from build123d import *

# Parameters (mm, degrees)
AUFSATZ_LINEAR_AUSTRAGEN1_DEPTH = 30
F_3_0_3_DURCHMESSER_BOHRUNG1_D  = 3
SCHNITT_LINEAR_AUSTRAGEN1_DEPTH = 4


with BuildPart() as part:
    # Skizze1 → Aufsatz-Linear austragen1 (new body)
    with BuildSketch(Plane.XY):
        with BuildLine():
            Line((-63.596153483, 25.865230167), (-58.344999569, 25.865230167))
            ThreePointArc((-58.344999569, 25.865230167), (-48.596153483, 34.665230167), (-38.847307398, 25.865230167))
            Line((-38.847307398, 25.865230167), (-34.847307398, 25.865230167))
            Line((-34.847307398, 25.865230167), (-34.176711032, 25.865230167))
            Line((-34.176711032, 25.865230167), (-33.778455993, 25.865230167))
            Line((-33.778455993, 25.865230167), (-33.778455993, 37.365230166))
            Line((-33.778455993, 37.365230166), (-34.847307398, 37.365230166))
            Line((-34.847307398, 37.365230166), (-48.596153483, 37.365230166))
            Line((-48.596153483, 37.365230166), (-63.596153483, 37.365230166))
            Line((-63.596153483, 37.365230166), (-63.596153483, 25.865230167))
        make_face()
    extrude(amount=-AUFSATZ_LINEAR_AUSTRAGEN1_DEPTH)

    # Ø3.0 (3) Durchmesser Bohrung1 (through all)
    with Locations(Plane(origin=(0, 37.365230166, 0), x_dir=(1, 0, 0), z_dir=(0, 1, 0))):
        with Locations((-36.847307398, 5), (-60.344999569, 5), (-60.344999569, 25), (-36.847307398, 25)):
            Hole(F_3_0_3_DURCHMESSER_BOHRUNG1_D / 2)

    # Skizze4 → Schnitt-Linear austragen1 (cut)
    with BuildSketch(Plane(origin=(0, 37.365230166, 0), x_dir=(1, 0, 0), z_dir=(0, 1, 0))):
        Polygon((-39.747307398, 26.674315781), (-39.747307398, 23.325684219), (-36.847307398, 21.651368439), (-33.947307398, 23.325684219), (-33.947307398, 26.674315781), (-36.847307398, 28.348631561), align=None)
        Polygon((-60.344999569, 28.348631561), (-63.244999569, 26.674315781), (-63.244999569, 23.325684219), (-60.344999569, 21.651368439), (-57.444999569, 23.325684219), (-57.444999569, 26.674315781), align=None)
        Polygon((-63.244999569, 6.674315781), (-63.244999569, 3.325684219), (-60.344999569, 1.651368439), (-57.444999569, 3.325684219), (-57.444999569, 6.674315781), (-60.344999569, 8.348631561), align=None)
        Polygon((-36.847307398, 8.348631561), (-39.747307398, 6.674315781), (-39.747307398, 3.325684219), (-36.847307398, 1.651368439), (-33.947307398, 3.325684219), (-33.947307398, 6.674315781), align=None)
    extrude(amount=-SCHNITT_LINEAR_AUSTRAGEN1_DEPTH, mode=Mode.SUBTRACT)


solid = part.part
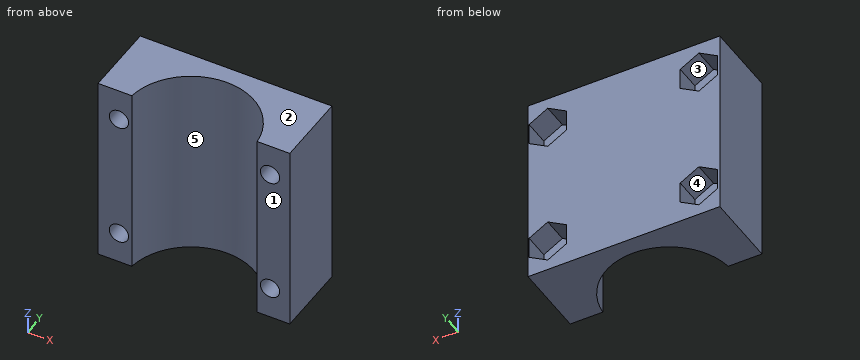
For this review, take the finished solid that the model builds, in its own axes (mm). Face numbers are marked on the shaded views. A direction names the side the tool comes from. Give positions to 0.01 mm unless a question says otherwise; leave off trailing zeros. Loops run counter-clockwise (first coordinate to the right, second up) from the corner with the lowest first, then second, coordinate; pieces in that order, holes last.
Item 1: Take a section at D-D, the plane x = -39.25. State the section outline as (y, z) points.
Item 2: Draft analysis for pull direction Z (two halves, no side actions). For the marked faces 1, 2 and 3, state which applies: +Z half, -Z half, draft (parallel to the pull), parting line (faces both ways), or undercut.
Item 3: Tool access review of the marked faces 4 and 5: name each direction out of +Z, -Z, +X, -X, +Y, -Y from which nothing blocks a thin tool from reaching the whole face with its end or side.
Item 4: For line 1 along Z through (x, y) = (-37, 27.25); line 2 along X through (y, z) = (30.25, -25) (3 decimals); line 3 along X through (y, z) = (32, -26), list the stretches that pass through material, from the lowest coordinate up.
Item 5: Insertion check: pin 1 (3 mm diameter, centred on x = -60.5, z = -24, fed in from +Y). The pin has a flat end and moves straight along its axis. Give the tip position at first contact, or say it passes through.
Item 6: Take a section at C-C, the plane z = -12. State the section outline as (x, y) points (3 decimals), and give its area (3 significant figures).
Item 7: Take a section at A-A, the plane z = -25. State the section outline as (x, y) points (3 decimals), and give its area (3 significant figures).
Item 8: Take a section at B-B, the plane y = 32. State the section outline as (x, z) points (3 decimals).
Calculated:
1. outline: (27.81, -30) - (37.37, -30) - (37.37, -26.96) - (33.37, -26.96) - (33.37, -23.04) - (37.37, -23.04) - (37.37, -6.96) - (33.37, -6.96) - (33.37, -3.04) - (37.37, -3.04) - (37.37, 0) - (27.81, 0) - close
2. face 1: draft
2. face 2: +Z half
2. face 3: undercut
3. face 4: +Y
3. face 5: +Z, -Z, -Y
4. line 1: z = -30 to -26.49, -23.51 to -6.49, -3.51 to 0
4. line 2: x = -63.596 to -61.845, -58.845 to -56.784, -40.408 to -38.347, -35.347 to -33.778
4. line 3: x = -63.6 to -61.46, -59.23 to -55.31, -41.88 to -37.97, -35.73 to -33.78
5. pin 1: stops at y = 33.37
6. outline: (-63.596, 25.865) - (-58.345, 25.865) arc R9.8 cw to (-38.847, 25.865) - (-33.778, 25.865) - (-33.778, 37.365) - (-63.596, 37.365) - close
6. area: 212 mm2
7. outline: (-63.596, 25.865) - (-61.845, 25.865) - (-61.845, 33.365) - (-63.245, 33.365) - (-63.245, 37.365) - (-63.596, 37.365) - close; (-58.845, 25.865) - (-58.345, 25.865) arc R9.8 cw to (-38.847, 25.865) - (-38.347, 25.865) - (-38.347, 33.365) - (-39.747, 33.365) - (-39.747, 37.365) - (-57.445, 37.365) - (-57.445, 33.365) - (-58.845, 33.365) - close; (-35.347, 25.865) - (-33.778, 25.865) - (-33.778, 37.365) - (-33.947, 37.365) - (-33.947, 33.365) - (-35.347, 33.365) - close
7. area: 120 mm2
8. outline: (-63.596, -30) - (-55.314, -30) - (-55.314, 0) - (-63.596, 0) - close; (-41.878, -30) - (-33.778, -30) - (-33.778, 0) - (-41.878, 0) - close; hole circle Ø3 at (-60.345, -25); hole circle Ø3 at (-60.345, -5); hole circle Ø3 at (-36.847, -25); hole circle Ø3 at (-36.847, -5)
